Check sheet for the modelled part. Datum: model origin and axes. Units: mm. Face numbers are marked on the shaded views. A direction names the side the tool comes from. Give positions to 0.01 mm unless a question says otherwise; leave off trailing zeros. Order: outer loops, then holes, each group sorted by start corner. A loop starts at its lowest first (then second) coordinate and runs counter-clockwise, first axis right, second up.
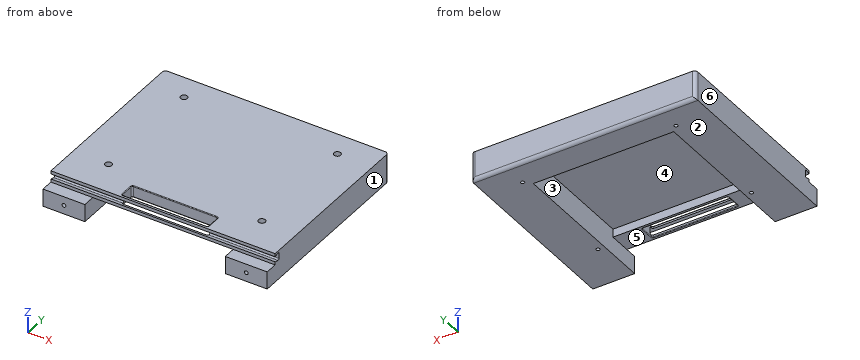
from build123d import *

# Parameters (mm, degrees)
SKETCH1_W           = 165.1
SKETCH1_H           = 100
BOSS_EXTRUDE1_DEPTH = 5
SKETCH4_W           = 165.1
SKETCH4_H           = 100
BOSS_EXTRUDE2_DEPTH = 3.5
SKETCH10_W          = 165.1
SKETCH10_H          = 8.5
BOSS_EXTRUDE4_DEPTH = 17
SKETCH11_W          = 103.4
SKETCH11_H          = 90.9
CUT_EXTRUDE6_DEPTH  = 6
SKETCH12_W          = 165.1
SKETCH12_H          = 13.05
BOSS_EXTRUDE5_DEPTH = 12.95
SKETCH13_W          = 165.1
SKETCH13_H          = 21.45
BOSS_EXTRUDE6_DEPTH = 9.75
SKETCH14_W          = 30.85
SKETCH14_H          = 115.7
BOSS_EXTRUDE7_DEPTH = 12.95
SKETCH15_R          = 1.35
CUT_EXTRUDE7_DEPTH  = 8.65
SKETCH16_R          = 2.5
CUT_EXTRUDE8_DEPTH  = 146.84584686
FILLET1_R           = 2.5
SKETCH17_W          = 165.1
SKETCH17_H          = 8.5
BOSS_EXTRUDE9_DEPTH = 2.75
CUT_EXTRUDE9_DEPTH  = 205.50252088
SKETCH21_R          = 1.35
CUT_EXTRUDE10_DEPTH = 17.5
SKETCH22_W          = 63.4
SKETCH22_H          = 11.8
CUT_EXTRUDE11_DEPTH = 10
FILLET2_R           = 1
FILLET3_R           = 0.5


with BuildPart() as part:
    # Sketch1 → Boss-Extrude1 (new body)
    with BuildSketch(Plane.XY):
        with Locations((0, -40.801949153)):
            Rectangle(SKETCH1_W, SKETCH1_H)
    extrude(amount=BOSS_EXTRUDE1_DEPTH)

    # Sketch4 → Boss-Extrude2 (add)
    with BuildSketch(Plane(origin=(0, 0, 0), x_dir=(-1, 0, 0), z_dir=(0, 0, -1))):
        with Locations((0, -40.801949153)):
            Rectangle(SKETCH4_W, SKETCH4_H)
    extrude(amount=BOSS_EXTRUDE2_DEPTH)

    # Sketch10 → Boss-Extrude4 (add)
    with BuildSketch(Plane.XZ.offset(90.801949153)):
        with Locations((0, 0.75)):
            Rectangle(SKETCH10_W, SKETCH10_H)
    extrude(amount=BOSS_EXTRUDE4_DEPTH)

    # Sketch11 → Cut-Extrude6 (cut)
    with BuildSketch(Plane(origin=(0, 0, -3.5), x_dir=(-1, 0, 0), z_dir=(0, 0, -1))):
        with Locations((0, -49.301949153)):
            Rectangle(SKETCH11_W, SKETCH11_H)
    extrude(amount=-CUT_EXTRUDE6_DEPTH, mode=Mode.SUBTRACT)

    # Sketch12 → Boss-Extrude5 (add)
    with BuildSketch(Plane(origin=(0, 0, -3.5), x_dir=(-1, 0, 0), z_dir=(0, 0, -1))):
        with Locations((0, 2.673050847)):
            Rectangle(SKETCH12_W, SKETCH12_H)
    extrude(amount=BOSS_EXTRUDE5_DEPTH)

    # Sketch13 → Boss-Extrude6 (add)
    with BuildSketch(Plane(origin=(0, 9.198050847, 0), x_dir=(1, 0, 0), z_dir=(0, 1, 0))):
        with Locations((0, 5.725)):
            Rectangle(SKETCH13_W, SKETCH13_H)
    extrude(amount=BOSS_EXTRUDE6_DEPTH)

    # Sketch14 → Boss-Extrude7 (add)
    with BuildSketch(Plane(origin=(0, 0, -3.5), x_dir=(-1, 0, 0), z_dir=(0, 0, -1))):
        Polygon((-51.7, -106.501949153), (-51.7, -119.551949153), (-82.55, -119.551949153), (-82.55, -3.851949153), (-51.7, -3.851949153), align=None)
        with Locations((67.125, -61.701949153)):
            Rectangle(SKETCH14_W, SKETCH14_H)
    extrude(amount=BOSS_EXTRUDE7_DEPTH)

    # Sketch15 → Cut-Extrude7 (cut)
    with BuildSketch(Plane(origin=(0, 0, -16.45), x_dir=(-1, 0, 0), z_dir=(0, 0, -1))):
        with Locations((56.3625, -85.271949153)):
            Circle(SKETCH15_R)
        with Locations((56.3625, 0.810550847)):
            Circle(SKETCH15_R)
        with Locations((-56.5625, 0.810550847)):
            Circle(SKETCH15_R)
        with Locations((-56.5625, -85.271949153)):
            Circle(SKETCH15_R)
    extrude(amount=-CUT_EXTRUDE7_DEPTH, mode=Mode.SUBTRACT)

    # Sketch16 → Cut-Extrude8 (cut, through all)
    with BuildSketch(Plane(origin=(0, 0, -7.8), x_dir=(-1, 0, 0), z_dir=(0, 0, -1))):
        with Locations((56.3625, 0.810550847)):
            Circle(SKETCH16_R)
        with Locations((-56.5625, 0.810550847)):
            Circle(SKETCH16_R)
        with Locations((-56.5625, -85.271949153)):
            Circle(SKETCH16_R)
        with Locations((56.3625, -85.271949153)):
            Circle(SKETCH16_R)
    extrude(amount=-CUT_EXTRUDE8_DEPTH, mode=Mode.SUBTRACT)

    # Fillet1
    fillet1_edges = [part.edges().sort_by_distance(p)[0] for p in [
        (-82.55, 18.948050847, -5.725),
        (82.55, 18.948050847, -5.725),
        (0, 18.948050847, -16.45),
    ]]
    fillet(fillet1_edges, radius=FILLET1_R)

    # Sketch17 → Boss-Extrude9 (add)
    with BuildSketch(Plane.XZ.offset(107.801949153)):
        with Locations((0, 0.75)):
            Rectangle(SKETCH17_W, SKETCH17_H)
    extrude(amount=BOSS_EXTRUDE9_DEPTH)

    # Sketch20 → Cut-Extrude9 (cut, through all)
    with BuildSketch(Plane(origin=(82.55, 0, 0), x_dir=(0, 0, -1), z_dir=(1, 0, 0))):
        with BuildLine():
            Line((1.155291427, -110.551949153), (2.030698282, -107.284886293))
            ThreePointArc((2.030698282, -107.284886293), (1.875383044, -106.504063866), (1.161365038, -106.151949153))
            Line((1.161365038, -106.151949153), (-2.661365038, -106.151949153))
            ThreePointArc((-2.661365038, -106.151949153), (-3.375383044, -106.504063866), (-3.530698282, -107.284886293))
            Line((-3.530698282, -107.284886293), (-2.655291427, -110.551949153))
            Line((-2.655291427, -110.551949153), (1.155291427, -110.551949153))
        make_face()
    extrude(amount=-CUT_EXTRUDE9_DEPTH, mode=Mode.SUBTRACT)

    # Sketch21 → Cut-Extrude10 (cut)
    with BuildSketch(Plane.XZ.offset(119.551949153)):
        with Locations(Location((-67.125, -9.975, 0), (0, 0, 270))):
            Circle(SKETCH21_R)
        with Locations(Location((67.125, -9.975, 0), (0, 0, 270))):
            Circle(SKETCH21_R)
    extrude(amount=-CUT_EXTRUDE10_DEPTH, mode=Mode.SUBTRACT)

    # Sketch22 → Cut-Extrude11 (cut)
    with BuildSketch(Plane(origin=(0, 0, -3.5), x_dir=(-1, 0, 0), z_dir=(0, 0, -1))):
        with Locations((0, -102.651949153)):
            Rectangle(SKETCH22_W, SKETCH22_H)
    extrude(amount=-CUT_EXTRUDE11_DEPTH, mode=Mode.SUBTRACT)

    # Fillet2
    fillet2_edges = [part.edges().sort_by_distance(p)[0] for p in [
        (31.7, -96.751949153, 0.75),
        (-31.7, -108.551949153, 4.095594906),
        (-31.7, -108.551949153, -2.595594906),
        (31.7, -108.551949153, 4.095594906),
        (31.7, -108.551949153, -2.595594906),
        (-31.7, -96.751949153, 0.75),
    ]]
    fillet(fillet2_edges, radius=FILLET2_R)

    # Fillet3
    fillet3_edges = [part.edges().sort_by_distance(p)[0] for p in [
        (31.407106781, -108.259055934, 5),
        (31.7, -102.651949153, 5),
        (31.407106781, -97.044842371, 5),
        (31.407106781, -97.044842371, -3.5),
        (0, -96.751949153, 5),
        (0, -96.751949153, -3.5),
        (-31.407106781, -97.044842371, 5),
        (-31.407106781, -97.044842371, -3.5),
        (-31.7, -102.651949153, 5),
        (-31.407106781, -108.259055934, 5),
        (0, -108.551949153, 5),
        (-31.407106781, -108.259055934, -3.5),
        (31.407106781, -108.259055934, -3.5),
    ]]
    fillet(fillet3_edges, radius=FILLET3_R)


solid = part.part
1) Section check A-A, the plane x = 1.5. Record the cut outline in (y, z), then the cut area to 3 significant figures.
Recorded:
outline: (-110.55, -3.5) - (-109.05, -3.5) arc R0.5 ccw to (-108.55, -3) - (-108.55, -1.69) - (-110.55, -1.16) - close; (-110.55, 2.66) - (-108.55, 3.19) - (-108.55, 4.5) arc R0.5 ccw to (-109.05, 5) - (-110.55, 5) - close; (-96.75, -3) arc R0.5 ccw to (-96.25, -3.5) - (-94.75, -3.5) - (-94.75, 2.5) - (-3.85, 2.5) - (-3.85, -16.45) - (16.45, -16.45) arc R2.5 ccw to (18.95, -13.95) - (18.95, 5) - (-96.25, 5) arc R0.5 ccw to (-96.75, 4.5) - close
area: 740 mm2
2) Section check C-C, the plane x = -43.5. Record the cut outline in (y, z), then the cut area to 3 significant figures.
Recorded:
outline: (-110.55, -3.5) - (-94.75, -3.5) - (-94.75, 2.5) - (-3.85, 2.5) - (-3.85, -16.45) - (16.45, -16.45) arc R2.5 ccw to (18.95, -13.95) - (18.95, 5) - (-110.55, 5) - (-110.55, 2.66) - (-107.28, 3.53) arc R0.9 cw to (-106.15, 2.66) - (-106.15, -1.16) arc R0.9 cw to (-107.28, -2.03) - (-110.55, -1.16) - close
area: 828 mm2
3) Section check B-B, the plane y = -17.5. Record the cut outline in (x, z), then the cut area to 3 significant figures.
Recorded:
outline: (-82.55, -16.45) - (-51.7, -16.45) - (-51.7, 2.5) - (51.7, 2.5) - (51.7, -16.45) - (82.55, -16.45) - (82.55, 5) - (-82.55, 5) - close
area: 1,580 mm2
4) Draft check along X on the marked faces 1, 2, 3 and 4. Enter one of: +X half, -X half, draft (parallel to the pull), parting line (faces both ways), or undercut.
Recorded:
face 1: +X half
face 2: draft
face 3: undercut
face 4: undercut
5) Material ranges on L1, parallel to X at y = -46.5, z = 0.25; L2, parallel to Y at x = 57.5, z = 1; L3, parallel to Y at x = 1, z = -3.25, recorded low to high.
Recorded:
L1: x = -82.55 to -51.7, 51.7 to 82.55
L2: y = -106.15 to -87.59, -82.95 to -1.51, 3.13 to 18.95
L3: y = -110.55 to -108.62, -96.68 to -94.75, -3.85 to 18.95
6) Set-up check for the marked faces 5 and 6: record each of +Z, -Z, +X, -X, +Y, -Y from which the full face is reachable in a straight line by a thin tool's end or side.
Recorded:
face 5: -Z, -Y
face 6: +Z, -Z, -X, +Y, -Y
7) Depth check by flat-ended pin: pin 1 Ø2 at (x, z) = (-66.5, -10.5) entering from -Y; pin 2 Ø3 at (x, y) = (17.5, -32) entering from -Z; pin 3 Ø4 at (x, z) = (52, 1) entering from -Y; pin 4 Ø3 at (x, z) = (-49.5, 0.5) entering from -Y. Enter the tip coordinate at first touch or a pass-through.
Recorded:
pin 1: stops at y = -119.55
pin 2: stops at z = 2.5
pin 3: stops at y = -110.55
pin 4: stops at y = -106.15
